The listing builds one solid part. Answer for the finished solid, in the listing's coordinates (mm). Give positions to 0.01 mm unless a question says otherwise; leave off trailing zeros. Write each loop counter-clockwise with the first axis right and the second up, starting at its lowest first coordinate (ties: lowest second). Pieces come first, ordered by that corner, then holes. Notation, with made-up numbers: M 27,17 L 49,17 A8 ccw 49,24 Z; hole C 22,-25.5 d8. An arc over 180 degrees is marked long. Answer as a JSON object with one key per item and string values.
```python
from build123d import *

# Parameters (mm, degrees)
SKETCH1_R           = 10
BOSS_EXTRUDE1_DEPTH = 75
DOME2_FACE_RADIUS   = 10
DOME2_HEIGHT        = 10
DOME3_FACE_RADIUS   = 10
DOME3_HEIGHT        = 10


with BuildPart() as part:
    # Sketch1 → Boss-Extrude1 (new body)
    with BuildSketch(Plane(origin=(0, 0, 0), x_dir=(1, 0, 0), z_dir=(0, 1, 0))):
        with Locations(Location((0, 0, 0), (0, 0, 270))):
            Circle(SKETCH1_R)
    extrude(amount=BOSS_EXTRUDE1_DEPTH)

    # Dome2: a dome of height H over a round flat face of radius A is a cap of a sphere of radius (A * A + H * H) / (2 * H)
    dome2_r = (DOME2_FACE_RADIUS * DOME2_FACE_RADIUS + DOME2_HEIGHT * DOME2_HEIGHT) / (2 * DOME2_HEIGHT)
    dome2_base = Plane((0, 75, 0), z_dir=(0, 1, 0))
    with Locations(dome2_base.offset(DOME2_HEIGHT - dome2_r)):
        dome2_ball = Sphere(dome2_r, mode=Mode.PRIVATE)
    add(split(dome2_ball, bisect_by=dome2_base, keep=Keep.TOP, mode=Mode.PRIVATE))

    # Dome3: a dome of height H over a round flat face of radius A is a cap of a sphere of radius (A * A + H * H) / (2 * H)
    dome3_r = (DOME3_FACE_RADIUS * DOME3_FACE_RADIUS + DOME3_HEIGHT * DOME3_HEIGHT) / (2 * DOME3_HEIGHT)
    dome3_base = Plane((0, 0, 0), z_dir=(0, -1, 0))
    with Locations(dome3_base.offset(DOME3_HEIGHT - dome3_r)):
        dome3_ball = Sphere(dome3_r, mode=Mode.PRIVATE)
    add(split(dome3_ball, bisect_by=dome3_base, keep=Keep.TOP, mode=Mode.PRIVATE))


solid = part.part
```
1. A cutting plane is placed at A-A, the plane x = 0. Give the vertices of the cut face in (y, z).
Verdict:
{"outline": "M 0,-10 L 75,-10 A10 ccw 75,10 L 0,10 A10 ccw Z"}
2. Flat-ended cylindrical pins translate along their axes: pin 1 (8 mm diameter, centred on x = -3.5, z = -0.5, fed in from +Y); pin 2 (5 mm diameter, centred on x = 7.5, y = 33.5, fed in from -Z); pin 3 (1.5 mm diameter, centred on y = 36.5, z = -7, fed in from +X); pin 4 (3 mm diameter, centred on x = -6.5, z = 3.5, fed in from -Y). Find the tip coordinate at first contact, or state that the pin passes through.
Verdict:
{"pin 1": "stops at y = 85", "pin 2": "stops at z = -8.66", "pin 3": "stops at x = 7.81", "pin 4": "stops at y = -8.09"}
3. Consider line 1 along Y through (x, z) = (-7.5, -2); line 2 along Y through (x, z) = (-5, 3); line 3 along X through (y, z) = (25.5, -8.5). Determine where each line is inside the solid, lowest interval first.
Verdict:
{"line 1": "y = -6.3 to 81.3", "line 2": "y = -8.12 to 83.12", "line 3": "x = -5.27 to 5.27"}
4. A cutting plane is placed at B-B, the plane y = 73.5. Give the vertices of the cut face in (x, z), plus the area to 3 significant figures.
Verdict:
{"outline": "C 0,0 d20", "area": "314 mm2"}
5. A cutting plane is placed at C-C, the plane z = -6.75. Give the vertices of the cut face in (x, y).
Verdict:
{"outline": "M -7.38,0 A7.38 ccw 7.38,0 L 7.38,75 A7.38 ccw -7.38,75 Z"}
